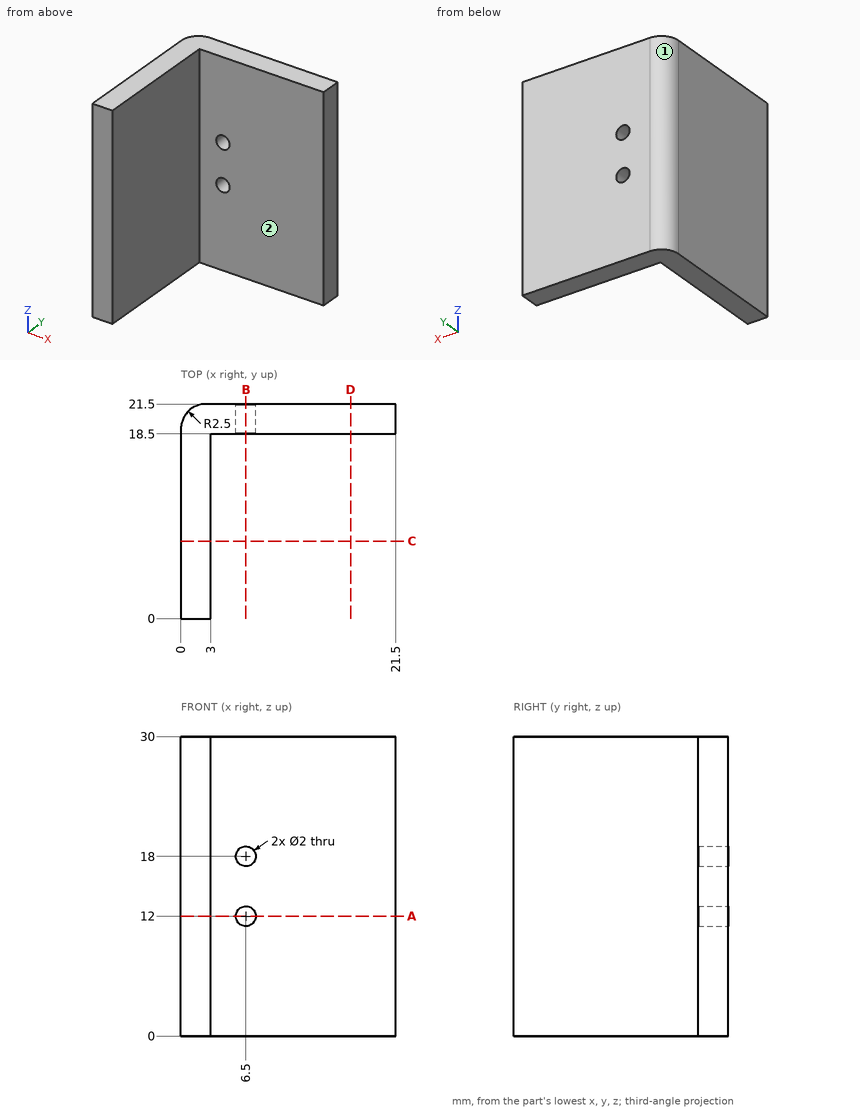
Answer from the drawing. Dimensions are ordinates in mm from the lowest x, y and z of the part. A direction names the side the tool comes from. Give positions to 0.01 mm unless a question says otherwise; leave off trailing zeros. Loops run counter-clockwise (first coordinate to the right, second up) from the corner with the lowest first, then second, coordinate; pieces in that order, holes last.
Item 1: The part is cut by section B-B (x = 6.5). Write down the section's boundary in (y, z).
Item 2: The part is cut by section A-A (z = 12). Write down the section's boundary in (x, y), and give its area (3 significant figures).
Item 3: For the marked faces 1 and 2, determine the directions among +Z, -Z, +X, -X, +Y, -Y from which every point of the face is accessible in a straight line to the end or side of a thin tool.
Item 4: The part is cut by section C-C (y = 7.75). Write down the section's boundary in (x, z).
Item 5: Each of these flat-tipped pins is pushed along its axis until it touches: pin 1 Ø1.5 at (y, z) = (5.5, 18) entering from +X; pin 2 Ø3 at (x, z) = (15, 5.5) entering from -Y. Where does it stop, or does it pass through?
Item 6: The part is cut by section D-D (x = 17). Write down the section's boundary in (y, z), and give its area (3 significant figures).
Item 7: Find the intervals of material crossed by line 1 along Z through (x, y) = (6.5, 20.85); line 2 along X through (y, z) = (15, 26.75); line 3 along Y through (x, z) = (4.5, 24.75), in increasing order.
Taken from the geometry:
1. outline: (18.5, 0) - (21.5, 0) - (21.5, 11) - (18.5, 11) - close; (18.5, 13) - (21.5, 13) - (21.5, 17) - (18.5, 17) - close; (18.5, 19) - (21.5, 19) - (21.5, 30) - (18.5, 30) - close
2. outline: (0, 0) - (3, 0) - (3, 18.5) - (5.5, 18.5) - (5.5, 21.5) - (2.5, 21.5) arc R2.5 ccw to (0, 19) - close; (7.5, 18.5) - (21.5, 18.5) - (21.5, 21.5) - (7.5, 21.5) - close
2. area: 113 mm2
3. face 1: +Z, -Z, -X, +Y
3. face 2: +Z, -Z, +X, -Y
4. outline: (0, 0) - (3, 0) - (3, 30) - (0, 30) - close
5. pin 1: stops at x = 3
5. pin 2: stops at y = 18.5
6. outline: (18.5, 0) - (21.5, 0) - (21.5, 30) - (18.5, 30) - close
6. area: 90.0 mm2
7. line 1: z = 0 to 11, 13 to 17, 19 to 30
7. line 2: x = 0 to 3
7. line 3: y = 18.5 to 21.5
